Work out the finished part from the listing and answer in its coordinate system (mm). A direction names the side the tool comes from. Give positions to 0.01 mm unless a question says otherwise; leave off trailing zeros. Loops run counter-clockwise (first coordinate to the right, second up) from the corner with the lowest first, then second, coordinate; pieces in that order, holes last. Notation, with made-up numbers: (31.25, 32) - (44.25, 32) arc R10 ccw to (44.25, 42) - close; hole circle Ø11 at (19.25, 86). An arc over 180 degrees is marked (long way). One line per question, with ' | ' between items.
from build123d import *

# Parameters (mm, degrees)
F1_DEPTH = 80
F2_W     = 10
F2_H     = 10
F3_DEPTH = 62.75
F4_DEPTH = 10
F5_R     = 2
F6_DEPTH = 25


with BuildPart() as f1:
    # F0 (on Top) → F1 (new body)
    with BuildSketch(Plane.XY):
        with BuildLine():
            ThreePointArc((0, 60), (21.2132034356, 51.2132034356), (30, 30))
            Line((30, 30), (30, 0))
            Line((30, 0), (33, 0))
            Line((33, 0), (33, 30))
            ThreePointArc((33, 30), (23.3345237792, 53.3345237792), (0, 63))
            Line((0, 63), (0, 60))
        make_face()
    extrude(amount=F1_DEPTH)

    # F2 (on Right) → F3 (cut)
    with BuildSketch(Plane.YZ):
        with Locations((58, 41.47)):
            Rectangle(F2_W, F2_H)
    extrude(amount=F3_DEPTH, mode=Mode.SUBTRACT)

    # F4 (add): a face of the model
    f4_faces = [f1.faces().sort_by_distance(p)[0] for p in [
        (21.4628397083, 53, 41.47),
    ]]
    extrude(f4_faces, amount=F4_DEPTH)

    # F5 (on face) → F6 (cut)
    with BuildSketch(Plane.YZ.offset(23.6643191324)):
        with Locations((58, 41.47)):
            Circle(F5_R)
    extrude(amount=-F6_DEPTH, mode=Mode.SUBTRACT)


solid = f1.part
1. Find section C-C on y = 58. Write down the section's boundary in (x, z), then the cut area to 3 significant figures.
Evaluation:
outline: (10.77, 0) - (17.46, 0) - (17.46, 36.47) - (10.77, 36.47) - close; (10.77, 46.47) - (17.46, 46.47) - (17.46, 80) - (10.77, 80) - close; (19.26, 36.47) - (23.66, 36.47) - (23.66, 39.47) - (19.26, 39.47) - close; (19.26, 43.47) - (23.66, 43.47) - (23.66, 46.47) - (19.26, 46.47) - close | area: 495 mm2
2. Find section B-B on x = 10. Write down the section's boundary in (y, z), then the cut area to 3 significant figures.
Evaluation:
outline: (58.28, 0) - (61.45, 0) - (61.45, 36.47) - (58.28, 36.47) - close; (58.28, 46.47) - (61.45, 46.47) - (61.45, 80) - (58.28, 80) - close | area: 221 mm2
3. Find section D-D on z = 60. Write down the section's boundary in (x, y), then the cut area to 3 significant figures.
Evaluation:
outline: (0, 60) arc R30 cw to (30, 30) - (30, 0) - (33, 0) - (33, 30) arc R33 ccw to (0, 63) - close | area: 238 mm2
4. Determine the mould class of faces 1 (the flat face through (33, 15, 39)), 2 (the flat face through (29, 41, 80)), 3 (the flat face through (29, 41, 0)), 4 (the cylindrical face through (21.5, 59.9, 42.1)) for opening direction Z: +Z half, -Z half, draft (parallel to the pull), parting line (faces both ways), or undercut.
Evaluation:
face 1: draft | face 2: +Z half | face 3: -Z half | face 4: undercut
5. Which of the six approach directions +Z, -Z, +X, -X, +Y, -Y give full straight-line access (tool end or side, diameter ignored) to faces 5 (the flat face through (10, 59, 36.47)), 6 (the flat face through (21, 59, 46.47)), 7 (the flat face through (23.664, 58, 39))?
Evaluation:
face 5: -X, +Y, -Y | face 6: +Z, +X, +Y | face 7: +Z, -Z, +X, +Y
6. Consider L1, parallel to Z at x = 22, y = 58; L2, parallel to X at y = 29, z = 71.5; L3, parallel to Y at x = 20, z = 56.5. Determine where each line is inside the solid, lowest interval first.
Evaluation:
L1: 36.47 to 39.47, 43.47 to 46.47 | L2: 30 to 33 | L3: 52.36 to 56.25
7. Flat-ended cylindrical pins translate along their axes: pin 1 (5 mm diameter, centred on y = 58, z = 41.47, fed in from -X); pin 2 (6 mm diameter, centred on y = 52, z = 22, fed in from -X); pin 3 (3.5 mm diameter, centred on x = 22, y = 58.5, fed in from +Z); pin 4 (3 mm diameter, centred on x = 8.5, y = 58.5, fed in from -Z). Find the tip coordinate at first contact, or state that the pin passes through.
Evaluation:
pin 1: x = 19.26 | pin 2: x = 16.58 | pin 3: z = 46.47 | pin 4: z = 0
8. Find section A-A on z = 41.47. Write down the section's boundary in (x, y).
Evaluation:
outline: (19.26, 53) arc R30 cw to (30, 30) - (30, 0) - (33, 0) - (33, 30) arc R33 ccw to (23.66, 53) - (23.66, 56) - (19.26, 56) - close; (19.26, 60) - (23.66, 60) - (23.66, 63) - (19.26, 63) - close
